CAD build for the part. Positions are in the model's coordinates, mm. Round coordinates to 2 decimals unless told otherwise and drop trailing zeros. Write each loop counter-clockwise with the first axis right and the second up, starting at its lowest first coordinate (ties: lowest second). Pieces come first, ordered by that corner, then holes. Notation, with made-up numbers: (4, 67.5) - (45, 67.5) arc R28 ccw to (45, 103.5) - close; hole circle Ø2 at (64.5, 20.5). An arc over 180 degrees is marked (long way). Answer in a Markdown table with one row per item.
Autodesk Inventor part; units mm, degrees
ref_plane "YZ Plane" through (0, 0, 0) normal (1, 0, 0) x (0, 1, 0)
ref_plane "XZ Plane" through (0, 0, 0) normal (0, 1, 0) x (-1, 0, 0)
ref_plane "XY Plane" through (0, 0, 0) normal (0, 0, 1) x (1, 0, 0)
sketch "Sketch1" plane through (0, 0, 0) normal (0, 1, 0) x (-1, 0, 0)
  circle A0 centre (0, 0) radius 177
  dimension "d0" = 354
extrude "Extrusion1" add sketch "Sketch1" along normal blind 5
sketch "Sketch2" plane through (0, 5, 0) normal (0, 1, 0) x (1, 0, 0)
  line L0 (0, 0) -> (153.2865, -88.5) construction
  circle A0 centre (0, 0) radius 177 construction
  line L1 (-177, 0) -> (177, 0) construction
  circle A1 centre (142.288, -82.15) radius 1.7
  line L2 (142.288, -82.15) -> (134.0391, -77.3875) construction
  circle A2 centre (142.288, -72.625) radius 1.7
  circle A3 centre (134.0391, -67.8625) radius 1.7
  circle A4 centre (125.7902, -72.625) radius 1.7
  circle A5 centre (125.7902, -82.15) radius 1.7
  circle A6 centre (134.0391, -86.9125) radius 1.7
  line L3 (0, 177) -> (0, -177) construction
  circle A7 centre (0, 0) radius 177 construction
  circle A8 centre (-142.288, -72.625) radius 1.7
  circle A9 centre (-125.7902, -72.625) radius 1.7
  circle A10 centre (-134.0391, -86.9125) radius 1.7
  circle A11 centre (0, 0) radius 177 construction
  circle A12 centre (142.288, 72.625) radius 1.7
  circle A13 centre (125.7902, 72.625) radius 1.7
  circle A14 centre (134.0391, 86.9125) radius 1.7
  circle A15 centre (-125.7902, 72.625) radius 1.7
  circle A16 centre (-142.288, 72.625) radius 1.7
  circle A17 centre (-134.0391, 86.9125) radius 1.7
  dimension "d3" = 30
  dimension "d4" = 3.4
  dimension "d5" = 12.7
  dimension "d6" = 9.525
  dimension "d9" = 360
extrude "Standoffs" cut sketch "Sketch2" against normal through all contours A2 | A4 | A6 | A8 | A9 | A10 | A12 | A13 | A14 | A15 | A16 | A17
sketch "Sketch3" plane through (0, 5, 0) normal (0, 1, 0) x (1, 0, 0)
  circle A0 centre (-127, 50.8) radius 10.16
  circle A1 centre (127, 50.8) radius 10.16
  circle A2 centre (0, 0) radius 177 construction
  circle A3 centre (0, 0) radius 177 construction
  line L0 (0, 0) -> (0, 177) construction
  line L1 (0, 0) -> (177, 0) construction
  line L2 (0, 0) -> (-177, 0) construction
  dimension "d13" = 20.32
  dimension "d14" = 20.32
  dimension "d19" = 127
  dimension "d20" = 127
  dimension "d21" = 50.8
  dimension "d22" = 50.8
extrude "Wires" cut sketch "Sketch3" against normal through all
sketch "Sketch4" plane through (0, 5, 0) normal (0, 1, 0) x (1, 0, 0)
  circle A0 centre (0, -141.44) radius 2.667
  circle A1 centre (0, 0) radius 177 construction
  line L0 (0, 0) -> (0, -177) construction
  line L1 (0, -177) -> (48.7641, -177) construction
  circle A2 centre (83.1363, -114.4274) radius 2.667
  circle A3 centre (-83.1363, -114.4274) radius 2.667
  circle A4 centre (134.5174, -43.7074) radius 2.667
  circle A5 centre (-134.5174, -43.7074) radius 2.667
  circle A6 centre (-34.3789, 137.1983) radius 2.667
  circle A7 centre (-101.628, 98.3718) radius 2.667
  line L2 (0, 0) -> (-34.3789, 137.1983) construction
  line L3 (0, 177) -> (0, -177) construction
  line L4 (-101.628, 98.3718) -> (0, 0) construction
  circle A8 centre (34.3789, 137.1983) radius 2.667
  circle A9 centre (101.628, 98.3718) radius 2.667
  dimension "d25" = 5.334
  dimension "d28" = 35.56
  dimension "d31" = 144
  dimension "d67" = 5.334
  dimension "d68" = 5.334
  dimension "d69" = 14.067
  dimension "d70" = 141.44
  dimension "d71" = 45.933
  dimension "d73" = 141.44
extrude "Zip Ties" cut sketch "Sketch4" against normal through all
sketch "Sketch5" plane through (0, 5, 0) normal (0, 1, 0) x (1, 0, 0)
  circle A0 centre (-63.5, 31.75) radius 1.7
  circle A1 centre (0, 0) radius 177 construction
  line L0 (-177, 0) -> (177, 0) construction
  line L1 (0, -177) -> (0, 177) construction
  circle A2 centre (63.5, 31.75) radius 1.7
  circle A3 centre (-63.5, -31.75) radius 1.7
  circle A4 centre (63.5, -31.75) radius 1.7
  dimension "d35" = 3.4
  dimension "d36" = 63.5
  dimension "d37" = 31.75
extrude "LiDAR" cut sketch "Sketch5" along normal through all both and the other way through all
sketch "Sketch6" plane through (0, 5, 0) normal (0, 1, 0) x (1, 0, 0)
  circle A0 centre (-17.145, 139.7) radius 1.7
  circle A1 centre (0, 0) radius 177 construction
  line L0 (-177, 0) -> (177, 0) construction
  line L1 (0, -196.4897) -> (0, 177) construction
  circle A2 centre (17.145, 139.7) radius 1.7
  dimension "d40" = 3.4
  dimension "d41" = 17.145
  dimension "d42" = 139.7
extrude "Astra Camera" cut sketch "Sketch6" against normal through all
sketch "Sketch7" plane through (0, 5, 0) normal (0, 1, 0) x (1, 0, 0)
  circle A0 centre (0, 0) radius 177 construction
  line L0 (-177, 0) -> (177, 0) construction
  line L1 (0, 177) -> (0, -177) construction
  circle A1 centre (-78.745, 44.45) radius 1.7
  circle A2 centre (-78.745, 123.61) radius 1.7
  circle A3 centre (78.745, 44.45) radius 1.7
  circle A4 centre (78.745, 123.61) radius 1.7
  dimension "d45" = 3.4
  dimension "d46" = 44.45
  dimension "d47" = 78.745
  dimension "d48" = 3.4
  dimension "d50" = 78.745
  dimension "d51" = 79.16
extrude "Display" cut sketch "Sketch7" against normal through all
sketch "Sketch8" plane through (0, 5, 0) normal (0, 1, 0) x (1, 0, 0)
  circle A0 centre (-10.795, 157.95) radius 1.7
  circle A1 centre (10.795, 157.95) radius 1.7
  circle A2 centre (0, 157.95) radius 3.175
  circle A3 centre (0, 0) radius 177 construction
  line L0 (0, 177) -> (46.0077, 177) construction
  line L1 (0, 177) -> (0, -177) construction
  dimension "d54" = 3.4
  dimension "d55" = 3.4
  dimension "d57" = 6.35
  dimension "d59" = 19.05
  dimension "d60" = 19.05
  dimension "d61" = 19.05
  dimension "d63" = 10.795
  dimension "d64" = 10.795
extrude "Arducam" cut sketch "Sketch8" against normal through all
equation "\"d0\" = robot_diameter"
equation "\"d1\" = hardboard_thickness"
equation "\"d4\" = m3_clearance"
equation "\"d14\" = d13"
equation "\"d22\" = d21"
equation "\"d67\" = d25"
equation "\"d68\" = d25"
equation "\"d73\" = d70"
equation "\"d35\" = m3_clearance"
equation "\"d40\" = m3_clearance"
equation "\"d45\" = m3_clearance"
equation "\"d48\" = d49"
equation "\"d50\" = d47"
equation "\"d54\" = m3_clearance"
equation "\"d55\" = d56"
equation "\"d60\" = d59"
equation "\"d61\" = d59"
equation "\"m3_heat_set_insert\" = 4"
equation "\"m3_clearance\" = 3.4"
equation "\"m3_heat_set_depth\" = 7"
equation "\"robot_diameter\" = 354"
equation "\"hardboard_thickness\" = 5"
equation "\"motor_centerline_height\" = 13"
properties part number "layer6_new"
Q1. Saw through at B-B on z = 66.5. List the corners of the cut face in (x, y), then the cut area to 3 significant figures.
Computed:
| item | result |
|---|---|
| outline | (-164.03, 0) - (164.03, 0) - (164.03, 5) - (-164.03, 5) - close |
| area | 1,640 mm2 |
Q2. Flat gauge pins, fed straight in: pin 1 (1.5 mm diameter, centred on y = 2.5, z = 82, fed in from -X); pin 2 (1 mm diameter, centred on y = 1.5, z = 134.5, fed in from +X); pin 3 (1 mm diameter, centred on x = -55.5, y = 0.5, fed in from +Z). Where does each tip first touch, or does it go through?
Computed:
| item | result |
|---|---|
| pin 1 | stops at x = -157.25 |
| pin 2 | stops at x = 115.64 |
| pin 3 | stops at z = 168.24 |
Q3. Saw through at A-A on z = -50.8. List the corners of the cut face in (x, y).
Computed:
| item | result |
|---|---|
| outline | (-169.55, 0) - (-137.16, 0) - (-137.16, 5) - (-169.55, 5) - close; (-116.84, 0) - (116.84, 0) - (116.84, 5) - (-116.84, 5) - close; (137.16, 0) - (169.55, 0) - (169.55, 5) - (137.16, 5) - close |
Q4. Saw through at C-C on x = 92.5. List the corners of the cut face in (y, z).
Computed:
| item | result |
|---|---|
| outline | (0, -150.91) - (5, -150.91) - (5, 150.91) - (0, 150.91) - close |
Q5. Pull direction Z, two halves, no side cores. Call faces 1 (the cylindrical face through (38.37, 2.46, 172.79)), 2 (the cylindrical face through (-137.15, 2.54, -51.25)), 3 (the flat face through (2, 0, 2)): released by +Z, released by -Z, zero draft, split by the parting line, or undercut.
Computed:
| item | result |
|---|---|
| face 1 | split by the parting line |
| face 2 | undercut |
| face 3 | zero draft |
Q6. Drill centre lines: line 1 (Z direction, x = 0, y = 3.15) (3 decimals); line 2 (X direction, y = 2.4, z = -87); line 3 (X direction, y = 1.55, z = 117.5). Where is each one in solid material? Low to high.
Computed:
| item | result |
|---|---|
| line 1 | z = -177 to -161.125, -154.775 to 138.773, 144.107 to 177 |
| line 2 | x = -154.14 to -135.74, -132.34 to 132.34, 135.74 to 154.14 |
| line 3 | x = -132.37 to 132.37 |
